Print and shaded views of the part. All mm, measured from the part's lowest x, y and z. A direction names the side the tool comes from. Round coordinates to 2 decimals unless told otherwise and drop trailing zeros. Loops run counter-clockwise (first coordinate to the right, second up) from the corner with the lowest first, then second, coordinate; pieces in that order, holes last. Notation, with made-up numbers: M -15,14.25 L 2,14.25 A8 ccw 2,27.25 Z; hole C -4.75,-20.75 d2. An arc over 180 degrees is marked long. One line per item, written item: value. Start each with the question number.
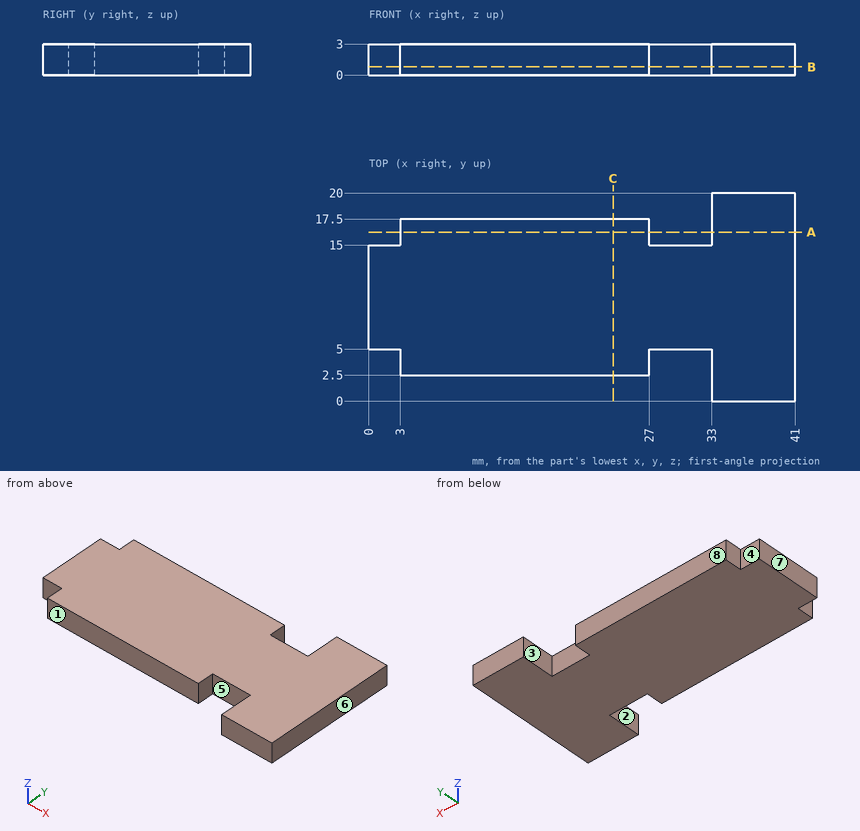
(1) Which spindle directions (+Z, -Z, +X, -X, +Y, -Y) get a long thin tool onto all of the face, cutting with end or side? Do the marked faces 1, 2, 3 and 4. Say none if no direction does.
(2) Slice it at C-C, the plane x = 23.5. List the corners of the cut face in (y, z).
(3) Probe L1, parallel to X at y = 4.5, z = 1.2; L2, parallel to Y at x = 20, z = 0.15; L3, parallel to Y at x = 32, z = 1.2. List the from-to ranges inside material, lowest first.
(4) Slice it at A-A, the plane y = 16.25. List the corners of the cut face in (x, z).
(5) Slice it at B-B, the plane z = 0.8. List the corners of the cut face in (x, y), and give its area (3 significant figures).
(6) Mould opens along X. For the marked faces 5, 6, 7 and 8 say: pulls with the +X half, pulls with the -X half, needs draft (parallel to the pull), parting line crosses it, or undercut.
(7) Flat gauge pins, fed straight in: P1, Ø0.8, axis at y = 16, z = 1.5, coming from the -X side; P2, Ø1.5, axis at x = 29, z = 1, coming from the -Y side; P3, Ø6, axis at x = 22.5, y = 8, coming from the -Z side; P4, Ø0.9, axis at x = 19.5, z = 1, coming from the -Y side. Where does each tip first touch, or does it go through?
Check result:
1. face 1: +Z, -Z, -X, -Y
1. face 2: +Z, -Z, -Y
1. face 3: +Z, -Z, +Y
1. face 4: +Z, -Z, -X, +Y
2. outline: M 2.5,0 L 17.5,0 L 17.5,3 L 2.5,3 Z
3. L1: x = 3 to 27, 33 to 41
3. L2: y = 2.5 to 17.5
3. L3: y = 5 to 15
4. outline: M 3,0 L 27,0 L 27,3 L 3,3 Z; M 33,0 L 41,0 L 41,3 L 33,3 Z
5. outline: M 0,5 L 3,5 L 3,2.5 L 27,2.5 L 27,5 L 33,5 L 33,0 L 41,0 L 41,20 L 33,20 L 33,15 L 27,15 L 27,17.5 L 3,17.5 L 3,15 L 0,15 Z
5. area: 610 mm^2
6. face 5: undercut
6. face 6: pulls with the +X half
6. face 7: pulls with the -X half
6. face 8: needs draft
7. P1: stops at x = 3
7. P2: stops at y = 5
7. P3: stops at z = 0
7. P4: stops at y = 2.5
